```python
from build123d import *

# Parameters (mm, degrees)
ESQUISSE1_R             = 0.5
BASE_EXTRUSION_DEPTH    = 3.2
ESQUISSE2_W             = 8
ESQUISSE2_H             = 0.5
BOSS_EXTRU_3_DEPTH      = 1.6
BOSS_EXTRU_MINCE1_DEPTH = 3.2
ESQUISSE4_R             = 0.5
ENL_V_MAT_EXTRU_1_DEPTH = 12.01944191
CONG_1_R                = 1.6


with BuildPart() as part:
    # Esquisse1 → Base-Extrusion (new, symmetric)
    with BuildSketch(Plane.XY):
        Circle(ESQUISSE1_R)
    extrude(amount=BASE_EXTRUSION_DEPTH, both=True)

    # Esquisse2 → Boss.-Extru.3 (add, symmetric)
    with BuildSketch(Plane.XY):
        with Locations((3.5, 0.74)):
            Rectangle(ESQUISSE2_W, ESQUISSE2_H)
    extrude(amount=BOSS_EXTRU_3_DEPTH, both=True)

    # Esquisse3 → Boss.-Extru.-Mince1 (add)
    with BuildSketch(Plane(origin=(7.5, 0, 0), x_dir=(0, 0, -1), z_dir=(1, 0, 0))):
        with BuildLine():
            Line((-2.1, 6.09), (-2.1, 1.99))
            ThreePointArc((-2.1, 1.99), (-1.807106781, 1.282893219), (-1.1, 0.99))
            Line((-1.1, 0.99), (1.1, 0.99))
            ThreePointArc((1.1, 0.99), (1.807106781, 1.282893219), (2.1, 1.99))
            Line((2.1, 1.99), (2.1, 6.09))
            Line((2.1, 6.09), (1.6, 6.09))
            Line((1.6, 6.09), (1.6, 1.99))
            ThreePointArc((1.6, 1.99), (1.453553391, 1.636446609), (1.1, 1.49))
            Line((1.1, 1.49), (-1.1, 1.49))
            ThreePointArc((-1.1, 1.49), (-1.453553391, 1.636446609), (-1.6, 1.99))
            Line((-1.6, 1.99), (-1.6, 6.09))
            Line((-1.6, 6.09), (-2.1, 6.09))
        make_face()
    extrude(amount=-BOSS_EXTRU_MINCE1_DEPTH)

    # Esquisse4 → Enlèv. mat.-Extru.1 (cut, through all)
    with BuildSketch(Plane.XY.offset(2.1)):
        with Locations((5.9, 4.49)):
            Circle(ESQUISSE4_R)
    extrude(amount=-ENL_V_MAT_EXTRU_1_DEPTH, mode=Mode.SUBTRACT)

    # Congé1
    cong_1_edges = [part.edges().sort_by_distance(p)[0] for p in [
        (7.5, 6.09, 1.85),
        (7.5, 6.09, -1.85),
        (4.3, 6.09, 1.85),
        (4.3, 6.09, -1.85),
    ]]
    fillet(cong_1_edges, radius=CONG_1_R - 0.0001)  # a hair under: the kernel refuses the full size


solid = part.part
```
Could you check a few things on this model? Use its own coordinates, in mm. A direction names the side the tool comes from. Round coordinates to 2 decimals unless told otherwise and drop trailing zeros. Write each loop counter-clockwise with the first axis right and the second up, starting at its lowest first coordinate (ties: lowest second). Pieces come first, ordered by that corner, then holes. Notation, with made-up numbers: M 44,29.5 L 60,29.5 A22 ccw 60,40.5 Z; hole C 74,-20.5 d11. An arc over 180 degrees is marked long. Answer in a Markdown table with one row per item. Add a question column.
Q1. Will these pins go through, and if not, where does the flat tip stop? pin 1 Ø2.5 at (x, y) = (5.5, 4) entering from -Z; pin 2 Ø1 at (x, y) = (6.5, 4.5) entering from +Z; pin 3 Ø1 at (x, z) = (3, 0.5) entering from +Y; pin 4 Ø2.5 at (x, z) = (5.5, -0.5) entering from +Y.
Q2. If I drill on line 1 (Z direction, x = 4.75, y = 3.5); line 2 (Z direction, x = 0.25, y = 0.75); line 3 (Y direction, x = 5.9, z = 1.95), over which ranges is the centre line in solid material (lowest first)? Write a range as from..to.
Q3. If we mould it in two halves opening along Y, with no side actions, what happens to faces 1 (the flat face through (0, 0, -3.2)), 2 (the cylindrical face through (6.362, 4.298, 1.854)), 3 (the cylindrical face through (4.76, 5.61, 1.85))? For each: +Y half, -Y half, draft (parallel to the pull), parting line (faces both ways), or undercut.
Q4. Imagine slicing it at B-B (y = 2.75). Please give me the cut outline in (x, z).
Q5. Imagine slicing it at D-D (x = 0). Please give me the cut outline in (y, z), then the cut area to 3 significant figures.
Q6. Imagine slicing it at A-A (z = -0.5). Please give me the cut outline in (x, y), then the cut area to 3 significant figures.
Q7. Imagine slicing it at C-C (x = 5.5). Please give me the cut outline in (y, z).
Q8. On a 3-axis mill with a long thin cutter (end or side, diameter ignored), from which of +Z, -Z, +X, -X, +Y, -Y can I reach the whole of each face in a straight line? I mean faces 4 (the flat face through (5.9, 3.6, -1.6)), 5 (the flat face through (0, 0, 3.2)). Say none if no direction works.
Values:
| question | item | result |
|---|---|---|
| 1 | pin 1 | z = -2.1 |
| 1 | pin 2 | z = 2.1 |
| 1 | pin 3 | y = 0.99 |
| 1 | pin 4 | y = 6.09 |
| 2 | line 1 | -2.1..-1.6, 1.6..2.1 |
| 2 | line 2 | -1.6..1.6 |
| 2 | line 3 | 1.46..3.99, 4.99..6.09 |
| 3 | face 1 | draft |
| 3 | face 2 | undercut |
| 3 | face 3 | +Y half |
| 4 | outline | M 4.3,-2.1 L 7.5,-2.1 L 7.5,-1.6 L 4.3,-1.6 Z; M 4.3,1.6 L 7.5,1.6 L 7.5,2.1 L 4.3,2.1 Z |
| 5 | outline | M -0.5,-3.2 L 0.5,-3.2 L 0.5,-1.6 L 0.99,-1.6 L 0.99,1.6 L 0.5,1.6 L 0.5,3.2 L -0.5,3.2 Z |
| 5 | area | 7.97 mm^2 |
| 6 | outline | M -0.5,0.49 L -0.1,0.49 A0.5 ccw long 0.1,0.49 L 7.5,0.49 L 7.5,1.49 L 4.3,1.49 L 4.3,0.99 L -0.5,0.99 Z |
| 6 | area | 6.38 mm^2 |
| 7 | outline | M 0.49,-1.6 L 0.99,-1.6 L 0.99,-1.1 A1 ccw 1.99,-2.1 L 4.19,-2.1 L 4.19,-1.6 L 1.99,-1.6 A0.5 cw 1.49,-1.1 L 1.49,1.1 A0.5 cw 1.99,1.6 L 4.19,1.6 L 4.19,2.1 L 1.99,2.1 A1 ccw 0.99,1.1 L 0.99,1.6 L 0.49,1.6 Z; M 4.79,-2.1 L 6.04,-2.1 L 6.04,-1.6 L 4.79,-1.6 Z; M 4.79,1.6 L 6.04,1.6 L 6.04,2.1 L 4.79,2.1 Z |
| 8 | face 4 | +X, -X, +Y |
| 8 | face 5 | +Z, +X, -X, +Y, -Y |
